Can you work these out from the drawing? Everything is in mm from the part's minimum corner. Give positions to 0.01 mm unless a question says otherwise; leave off trailing zeros. Write each loop counter-clockwise with the first axis right and the second up, starting at its lowest first coordinate (ties: lowest second). Pieces come first, ordered by that corner, then holes. Notation, with made-up numbers: M 43,64 L 67,64 A13 ccw 67,76 Z; hole C 42,1 d6. An arc over 180 degrees is marked long. One line per item, written item: value.
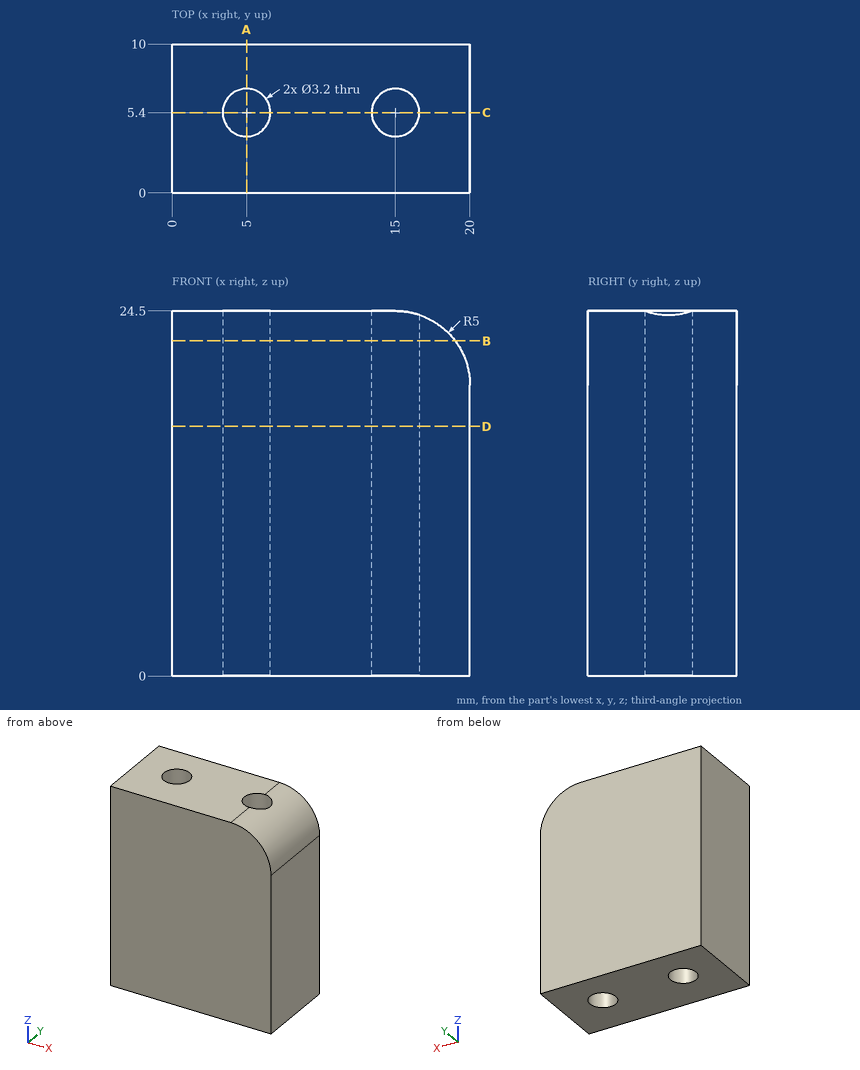
1) If we section it at D-D, the plane z = 16.75: Write out the boundary of the cut face in (x, y).
Outcome:
outline: M 0,0 L 20,0 L 20,10 L 0,10 Z; hole C 5,5.4 d3.2; hole C 15,5.4 d3.2
2) If we section it at A-A, the plane x = 5: Write out the boundary of the cut face in (y, z).
Outcome:
outline: M 0,0 L 3.8,0 L 3.8,24.5 L 0,24.5 Z; M 7,0 L 10,0 L 10,24.5 L 7,24.5 Z
3) Please list where these lines run through material, in increasing order: L1, parallel to X at y = 5.25, z = 17; L2, parallel to X at y = 5, z = 14; L3, parallel to Y at x = 16, z = 5. Write a range as from..to.
Outcome:
L1: x = 0..3.41, 6.59..13.41, 16.59..20
L2: x = 0..3.45, 6.55..13.45, 16.55..20
L3: y = 0..4.15, 6.65..10
4) If we section it at C-C, the plane y = 5.4: Write out the boundary of the cut face in (x, z).
Outcome:
outline: M 0,0 L 3.4,0 L 3.4,24.5 L 0,24.5 Z; M 6.6,0 L 13.4,0 L 13.4,24.5 L 6.6,24.5 Z; M 16.6,0 L 20,0 L 20,19.5 A5 ccw 16.6,24.24 Z
5) If we section it at B-B, the plane z = 22.5: Write out the boundary of the cut face in (x, y).
Outcome:
outline: M 0,0 L 19,0 L 19,10 L 0,10 Z; hole C 5,5.4 d3.2; hole C 15,5.4 d3.2
